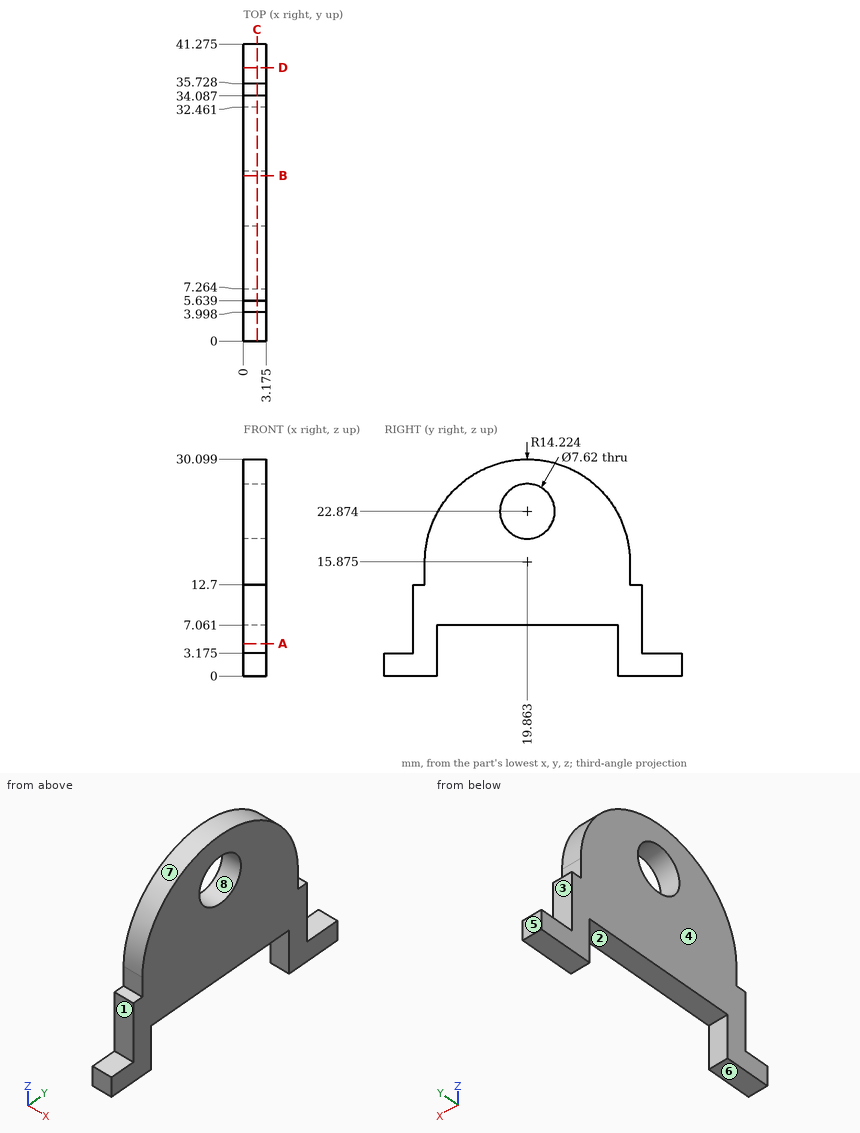
Drawing for the job (mm, zero at the part's lowest x, y, z). A direction names the side the tool comes from. Give positions to 0.01 mm unless a question says otherwise; leave off trailing zeros. Write each loop counter-clockwise with the first axis right and the second up, starting at its lowest first coordinate (ties: lowest second). Pieces come first, ordered by that corner, then holes. Notation, with made-up numbers: M 71.25,-6.75 L 110.25,-6.75 A20 cw 110.25,2.25 Z; hole C -17.5,-23 d11. An arc over 180 degrees is marked long. Return JSON: item names as keys, results as strings. Group by question number.
(1) Band-saw the part on D-D (y = 38). Give the cut face in (x, z) (1 decimal).
(2) Flat gauge pins, fed straight in: pin 1 Ø1.5 at (x, z) = (1, 19) entering from -Y; pin 2 Ø1 at (x, y) = (2, 2.5) entering from +Z (3 decimals); pin 3 Ø0.5 at (x, y) = (1, 35.5) entering from +Z. Where does each tip first touch, or does it go through?
(3) Mould opens along Z. For the marked faces 5, 6, 7 and 8 say: pulls with the +Z half, pulls with the -Z half, needs draft (parallel to the pull), parting line crosses it, or undercut.
(4) Band-saw the part on B-B (y = 23). Give the cut face in (x, z) (1 decimal).
(5) Band-saw the part on C-C (x = 1.9). Give the cut face in (y, z) (1 decimal).
(6) 3-axis set-ups, long thin cutter, end or side, ignore diameter. For the marked faces 1, 2, 3 and 4: which of +Z, -Z, +X, -X, +Y, -Y reach the whole face in a straight line?
(7) Band-saw the part on A-A (z = 4.5). Give the cut face in (x, y) (1 decimal).
(8) Drill centre lines: L1, parallel to Y at x = 2.4, z = 4 (1 decimal); L2, parallel to Y at x = 1.7, z = 8; L3, parallel to Z at x = 2.9, y = 5. Where is each one in solid material? Low to high. Write a range as [from, to].
Entries:
{
 "1": {"outline": "M 0,0 L 3.2,0 L 3.2,3.2 L 0,3.2 Z"},
 "2": {"pin 1": "stops at y = 5.84", "pin 2": "stops at z = 3.175", "pin 3": "stops at z = 12.7"},
 "3": {"face 5": "needs draft", "face 6": "pulls with the -Z half", "face 7": "pulls with the +Z half", "face 8": "undercut"},
 "4": {"outline": "M 0,7.1 L 3.2,7.1 L 3.2,20.7 L 0,20.7 Z; M 0,25 L 3.2,25 L 3.2,29.7 L 0,29.7 Z"},
 "5": {"outline": "M 0,0 L 7.3,0 L 7.3,7.1 L 32.5,7.1 L 32.5,0 L 41.3,0 L 41.3,3.2 L 35.7,3.2 L 35.7,12.7 L 34.1,12.7 L 34.1,15.9 A14.2 ccw 5.6,15.9 L 5.6,12.7 L 4,12.7 L 4,3.2 L 0,3.2 Z; hole C 19.9,22.9 d7.6"},
 "6": {"face 1": "+Z, +X, -X, -Y", "face 2": "-Z, +X, -X", "face 3": "+Z, +X, -X, +Y", "face 4": "+Z, -Z, -X, +Y, -Y"},
 "7": {"outline": "M 0,4 L 3.2,4 L 3.2,7.3 L 0,7.3 Z; M 0,32.5 L 3.2,32.5 L 3.2,35.7 L 0,35.7 Z"},
 "8": {"L1": "y = [4, 7.3], [32.5, 35.7]", "L2": "y = [4, 35.73]", "L3": "z = [0, 12.7]"}
}
